```python
from build123d import *

# Parameters (mm, degrees)
SKETCH1_R           = 25
SKETCH1_R_2         = 23
BOSS_EXTRUDE1_DEPTH = 300
CUT_EXTRUDE1_DEPTH  = 51


with BuildPart() as part:
    # Sketch1 → Boss-Extrude1 (new body)
    with BuildSketch(Plane.XY):
        Circle(SKETCH1_R)
        Circle(SKETCH1_R_2, mode=Mode.SUBTRACT)
    extrude(amount=BOSS_EXTRUDE1_DEPTH)

    # Sketch2 → Cut-Extrude1 (cut)
    with BuildSketch(Plane(origin=(0, 50, 0), x_dir=(1, 0, 0), z_dir=(0, 1, 0))):
        with BuildLine():
            Line((5, -10), (-5, -10))
            ThreePointArc((-5, -10), (-12.071067812, -12.928932188), (-15, -20))
            Line((-15, -20), (-15, -280))
            ThreePointArc((-15, -280), (-12.071067812, -287.071067812), (-5, -290))
            Line((-5, -290), (5, -290))
            ThreePointArc((5, -290), (12.071067812, -287.071067812), (15, -280))
            Line((15, -280), (15, -20))
            ThreePointArc((15, -20), (12.071067812, -12.928932188), (5, -10))
        make_face()
    extrude(amount=-CUT_EXTRUDE1_DEPTH, mode=Mode.SUBTRACT)


solid = part.part
```
For this review, take the finished solid that the model builds, in its own axes (mm). A direction names the side the tool comes from. Coordinates: 2 decimals unless noted, no trailing zeros. Write each loop counter-clockwise with the first axis right and the second up, starting at its lowest first coordinate (ties: lowest second). Pieces come first, ordered by that corner, then holes.
(1) Wall thickness on probe 1 along X at (y, z) = (-1, 120); probe 2 along Y at (x, z) = (0, 156); probe 3 along X at (y, z) = (6, 72.5): over which ranges is each line inside the solid? List them lowest first.
(2) Add section D-D on z = 152. Give the boundary of the cut face in (x, y).
(3) The part is to be moulded in two halves that separate along Y. For faces 1 (the face through (-5.42, -24.406, 147.9)), 2 (the face through (22.1, -7.3, 0)), 3 (the face through (-4.986, -22.453, 147.9)), say which applies: +Y half, -Y half, draft (parallel to the pull), parting line (faces both ways), or undercut.
(4) Tool access review of faces 4 (the face through (22.1, -7.3, 300)), 5 (the face through (-12.495, 20.982, 286.621)): name each direction out of +Z, -Z, +X, -X, +Y, -Y from which nothing blocks a thin tool from reaching the whole face with its end or side.
(5) Add section C-C on x = -19.5. Give the boundary of the cut face in (y, z).
(6) For pin 1 Ø2 at (y, z) = (19, 146.5) entering from +X; pin 2 Ø2 at (x, z) = (-12.5, 199.5) entering from -Y; pin 3 Ø5 at (y, z) = (-20, 153.5) entering from +X, all flat-tipped, find the tip position at first contact; note any pin that passes through.
(7) Add section B-B on x = 0. Give the boundary of the cut face in (y, z), then the cut area to 3 significant figures.
(8) Add section A-A on y = 0. Give the boundary of the cut face in (x, z), then the cut area to 3 significant figures.
Answer sheet:
1. probe 1: x = -24.98 to -22.98, 22.98 to 24.98
1. probe 2: y = -25 to -23
1. probe 3: x = -24.27 to -22.2, 22.2 to 24.27
2. outline: (-15, 17.44) - (-15, 20) arc R25 ccw (long way) to (15, 20) - (15, 17.44) arc R23 cw (long way) to start
3. face 1: parting line
3. face 2: draft
3. face 3: undercut
4. face 4: +Z, +X, -X, +Y, -Y
4. face 5: +Y
5. outline: (-15.64, 0) - (-12.2, 0) - (-12.2, 300) - (-15.64, 300) - close; (12.2, 0) - (15.64, 0) - (15.64, 300) - (12.2, 300) - close
6. pin 1: stops at x = 17.35
6. pin 2: stops at y = -22.2
6. pin 3: stops at x = 17.85
7. outline: (-25, 0) - (-23, 0) - (-23, 300) - (-25, 300) - close; (23, 0) - (25, 0) - (25, 10) - (23, 10) - close; (23, 290) - (25, 290) - (25, 300) - (23, 300) - close
7. area: 640 mm2
8. outline: (-25, 0) - (-23, 0) - (-23, 300) - (-25, 300) - close; (23, 0) - (25, 0) - (25, 300) - (23, 300) - close
8. area: 1,200 mm2
